The listing builds one solid part. Answer for the finished solid, in the listing's coordinates (mm). A direction names the side the tool comes from. Give positions to 0.01 mm unless a question says otherwise; leave off trailing zeros. Loops run counter-clockwise (first coordinate to the right, second up) from the corner with the lowest first, then second, coordinate; pieces in that order, holes last. Notation, with made-up numbers: (-38.75, -21) - (-34.75, -21) arc R23 ccw to (-34.75, -5) - close; hole circle Ø4 at (-6.5, 39). An arc over 180 degrees is marked (long way). One line per item, written item: value. Start each with the question number.
from build123d import *

# Parameters (mm, degrees)
F0_DEPTH = 38.1
F1_R     = 31.75
F1_R_2   = 12.7
F4_DEPTH = 25.4
F2_R     = 5.08


with BuildPart() as f0:
    # F3 (on Front) → F0 (new body)
    with BuildSketch(Plane.XZ):
        with BuildLine():
            ThreePointArc((12.7, 49.186888), (40.160926, 31.10852), (50.8, 0))
            ThreePointArc((50.8, 0), (40.160926, -31.10852), (12.7, -49.186888))
            Line((12.7, -49.186888), (107.95, -24.593444))
            ThreePointArc((107.95, -24.593444), (76.2, 0), (107.95, 24.593444))
            Line((107.95, 24.593444), (12.7, 49.186888))
        make_face()
        with BuildLine():
            ThreePointArc((12.7, -49.186888), (40.160926, -31.10852), (50.8, 0))
            ThreePointArc((50.8, 0), (40.160926, 31.10852), (12.7, 49.186888))
            ThreePointArc((12.7, 49.186888), (-50.8, 0), (12.7, -49.186888))
        make_face()
        with BuildLine():
            ThreePointArc((127, 0), (121.680463, 15.55426), (107.95, 24.593444))
            ThreePointArc((107.95, 24.593444), (76.2, 0), (107.95, -24.593444))
            ThreePointArc((107.95, -24.593444), (121.680463, -15.55426), (127, 0))
        make_face()
    extrude(amount=F0_DEPTH)

    # F1 (on face) → F4 (cut)
    with BuildSketch(Plane.XZ.offset(38.1)):
        Circle(F1_R)
        with Locations((101.6, 0)):
            Circle(F1_R_2)
    extrude(amount=-F4_DEPTH, mode=Mode.SUBTRACT)

    # F2
    f2_edges = [f0.edges().sort_by_distance(p)[0] for p in [
        (-31.75, -38.1, 0),
        (88.9, -38.1, 0),
        (60.325, -38.1, 36.890166),
    ]]
    fillet(f2_edges, radius=F2_R)


solid = f0.part
1. Find the intervals of material crossed by L1, parallel to Z at x = 0, y = -27.75; L2, parallel to Z at x = 101.6, y = -17; L3, parallel to Y at x = -19, z = 11.5, in increasing order. Write a range as [from, to].
2. A cutting plane is placed at B-B (y = -6). Determine the outline of the cut face in (x, z), plus the area to 3 significant figures.
3. Flat-ended cylindrical pins translate along their axes: pin 1 (10 mm diameter, centred on x = -0.5, y = -14.5, fed in from -Z); pin 2 (20.5 mm diameter, centred on x = 101.6, z = 0, fed in from -Y); pin 3 (12 mm diameter, centred on x = 85, y = -15, fed in from +Z). Find the tip coordinate at first contact, or state that the pin passes through.
4. A cutting plane is placed at A-A (y = -18.5). Determine the outline of the cut face in (x, z), plus the area to 3 significant figures.
5. Determine the mould class of faces 1 (the cylindrical face through (113.714, -23.002, 3.815)), 2 (the flat face through (37, -38.1, 1)), 3 (the flat face through (59.66, -16.28, -37.06)) for opening direction Z: released by +Z, released by -Z, zero draft, split by the parting line, or undercut.
6. For faces 4 (the flat face through (101, -12.7, 0)), 5 (the cylindrical face through (60.61, -36.65, -35.24)), determine the directions among +Z, -Z, +X, -X, +Y, -Y from which every point of the face is accessible in a straight line to the end or side of a thin tool.
Results below:
1. L1: z = [-50.8, -31.75], [31.75, 50.8]
1. L2: z = [-26.23, -12.7], [12.7, 26.23]
1. L3: y = [-12.7, 0]
2. outline: (12.7, -49.19) - (107.95, -24.59) arc R25.4 ccw to (107.95, 24.59) - (12.7, 49.19) arc R50.8 ccw (long way) to start
2. area: 13,100 mm^2
3. pin 1: stops at z = -50.8
3. pin 2: stops at y = -12.7
3. pin 3: stops at z = 32.07
4. outline: (12.7, -49.19) - (107.95, -24.59) arc R25.4 ccw to (107.95, 24.59) - (12.7, 49.19) arc R50.8 ccw (long way) to start; hole circle Ø63.5 at (0, 0); hole circle Ø25.4 at (101.6, 0)
4. area: 9,380 mm^2
5. face 1: undercut
5. face 2: zero draft
5. face 3: released by -Z
6. face 4: -Y
6. face 5: -Z, +X, -Y
